```python
from build123d import *

# Parameters (mm, degrees)
BOSS_EXTRUDE1_DEPTH = 75
SHELL4_START        = 5
SHELL4_DEPTH        = 70


# Read off the part's stored shape, not the designer's step: Shell4
with BuildPart() as part:
    # Sketch1 → Boss-Extrude1 (new body)
    with BuildSketch(Plane(origin=(0, 0, 0), x_dir=(1, 0, 0), z_dir=(0, 1, 0))):
        with BuildLine():
            Line((16.770509831, 15), (16.770509831, -15))
            ThreePointArc((16.770509831, -15), (-22.5, 0), (16.770509831, 15))
        make_face()
    extrude(amount=BOSS_EXTRUDE1_DEPTH)

    # Shell4 outline → Shell4 (cut)
    with BuildSketch(Plane(origin=(0, 0, 0), x_dir=(1, 0, 0), z_dir=(0, 1, 0)).offset(SHELL4_START)):
        with BuildLine():
            ThreePointArc((6.770509831, 20.406131349), (-21.5, 0), (6.770509831, -20.406131349))
            Line((6.770509831, -20.406131349), (6.770509831, 20.406131349))
        make_face()
    extrude(amount=SHELL4_DEPTH, mode=Mode.SUBTRACT)


solid = part.part
```
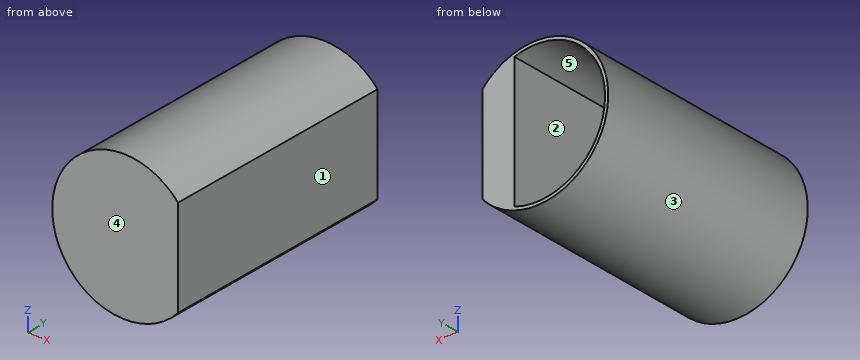
Could you check a few things on this model? Use its own coordinates, in mm. Face numbers are marked on the shaded views. A direction names the side the tool comes from. Round coordinates to 2 decimals unless told otherwise and drop trailing zeros. Loops run counter-clockwise (first coordinate to the right, second up) from the corner with the lowest first, then second, coordinate; pieces in that order, holes last. Notation, with made-up numbers: M 46,65 L 100,65 A30 ccw 100,96 Z; hole C 12,31.25 d11. An arc over 180 degrees is marked long. Write item = value, one per line.
1. Which directions (+Z, -Z, +X, -X, +Y, -Y) give clear straight access to the entire face, cutting with the end or side of a thin tool? Please do the marked faces 1 and 2.
Results below:
face_1 = +Z, -Z, +X, +Y, -Y
face_2 = +Y
2. I want a section at B-B, the plane z = 0. Write out the boundary of the cut face in (x, y), and give its area (3 significant figures).
Results below:
outline = M -22.5,0 L 16.77,0 L 16.77,75 L 6.77,75 L 6.77,5 L -21.5,5 L -21.5,75 L -22.5,75 Z
area = 966 mm²
3. I want a section at A-A, the plane x = 0. Write out the boundary of the cut face in (y, z), and give its area (3 significant figures).
Results below:
outline = M 0,-22.5 L 75,-22.5 L 75,-21.5 L 5,-21.5 L 5,21.5 L 75,21.5 L 75,22.5 L 0,22.5 Z
area = 365 mm²
4. Thinking about a two-plate mould opening in Z: for the marked faces 3, 4 and 5, which applies, +Z half, -Z half, draft (parallel to the pull), parting line (faces both ways), or undercut?
Results below:
face_3 = parting line
face_4 = draft
face_5 = undercut
5. I need wall thicknesses on probe 1 along X at (y, z) = (22, 0); probe 2 along Z at (x, y) = (0, 35); probe 3 along Y at (x, z) = (0.5, 13). Which ranges of each line are inside material? Lowest first, please.
Results below:
probe_1 = -22.5 to -21.5, 6.77 to 16.77
probe_2 = -22.5 to -21.5, 21.5 to 22.5
probe_3 = 0 to 5
6. Will these pins go through, and if not, where does the flat tip stop? P1, Ø20.5, axis at y = 29.5, z = -8, coming from the -X side; P2, Ø1, axis at y = 34, z = -8.5, coming from the -X side; P3, Ø8, axis at x = -13, y = 37.5, coming from the +Z side.
Results below:
P1 = -22.5
P2 = -21.03
P3 = 20.62
7. I want a section at C-C, the plane y = 29. Write out the boundary of the cut face in (x, z), and give its area (3 significant figures).
Results below:
outline = M 16.77,-15 L 16.77,15 A22.5 ccw long Z; hole M 6.77,-20.41 L 6.77,20.41 A21.5 ccw long Z
area = 460 mm²
